from build123d import *

# Parameters (mm, degrees)
SKETCH3_R             = 2.5
SKETCH3_R_2           = 1.5
BOSS_EXTRUDE2_DEPTH   = 14
BOSS_EXTRUDE2_2_DEPTH = 14
BOSS_EXTRUDE2_3_DEPTH = 14
BOSS_EXTRUDE2_4_DEPTH = 14
BOSS_EXTRUDE3_DEPTH   = 1.5
SKETCH5_R             = 1.5
CUT_EXTRUDE1_DEPTH    = 1.5
CUT_EXTRUDE2_DEPTH    = 1.5


with BuildPart() as part:
    # Sketch3 → Boss-Extrude2 (new body)
    with BuildSketch(Plane(origin=(0, 0, 0), x_dir=(1, 0, 0), z_dir=(0, 1, 0))):
        with Locations((-31, 18)):
            Circle(SKETCH3_R)
        with Locations((-31, 18)):
            Circle(SKETCH3_R_2, mode=Mode.SUBTRACT)
    extrude(amount=BOSS_EXTRUDE2_DEPTH)



with BuildPart() as body_2:
    # Sketch3 → Boss-Extrude2 2 (new body)
    with BuildSketch(Plane(origin=(0, 0, 0), x_dir=(1, 0, 0), z_dir=(0, 1, 0))):
        with Locations((31, 18)):
            Circle(SKETCH3_R)
        with Locations((31, 18)):
            Circle(SKETCH3_R_2, mode=Mode.SUBTRACT)
    extrude(amount=BOSS_EXTRUDE2_2_DEPTH)


with BuildPart() as body_3:
    # Sketch3 → Boss-Extrude2 3 (new body)
    with BuildSketch(Plane(origin=(0, 0, 0), x_dir=(1, 0, 0), z_dir=(0, 1, 0))):
        with Locations((31, -18)):
            Circle(SKETCH3_R)
        with Locations((31, -18)):
            Circle(SKETCH3_R_2, mode=Mode.SUBTRACT)
    extrude(amount=BOSS_EXTRUDE2_3_DEPTH)


with BuildPart() as body_4:
    # Sketch3 → Boss-Extrude2 4 (new body)
    with BuildSketch(Plane(origin=(0, 0, 0), x_dir=(1, 0, 0), z_dir=(0, 1, 0))):
        with Locations((-31, -18)):
            Circle(SKETCH3_R)
        with Locations((-31, -18)):
            Circle(SKETCH3_R_2, mode=Mode.SUBTRACT)
    extrude(amount=BOSS_EXTRUDE2_4_DEPTH)


with BuildPart() as part_1:
    add(part.part)

    add(body_2.part)  # Boss-Extrude3 merges body 2

    add(body_3.part)  # Boss-Extrude3 merges body 3

    add(body_4.part)  # Boss-Extrude3 merges body 4
    # Sketch4 → Boss-Extrude3 (add)
    with BuildSketch(Plane.XZ):
        with BuildLine():
            Line((-31, 20.5), (31, 20.5))
            ThreePointArc((31, 20.5), (32.767766953, 19.767766953), (33.5, 18))
            Line((33.5, 18), (33.5, -18))
            ThreePointArc((33.5, -18), (32.767766953, -19.767766953), (31, -20.5))
            Line((31, -20.5), (-31, -20.5))
            ThreePointArc((-31, -20.5), (-32.767766953, -19.767766953), (-33.5, -18))
            Line((-33.5, -18), (-33.5, 18))
            ThreePointArc((-33.5, 18), (-32.767766953, 19.767766953), (-31, 20.5))
        make_face()
    extrude(amount=BOSS_EXTRUDE3_DEPTH)

    # Sketch5 → Cut-Extrude1 (cut)
    with BuildSketch(Plane(origin=(0, 0, 0), x_dir=(1, 0, 0), z_dir=(0, 1, 0))):
        with Locations((31, 18)):
            Circle(SKETCH5_R)
        with Locations((-31, 18)):
            Circle(SKETCH5_R)
        with Locations((-31, -18)):
            Circle(SKETCH5_R)
        with Locations((31, -18)):
            Circle(SKETCH5_R)
    extrude(amount=-CUT_EXTRUDE1_DEPTH, mode=Mode.SUBTRACT)

    # Sketch6 → Cut-Extrude2 (cut)
    with BuildSketch(Plane(origin=(0, 0, 0), x_dir=(1, 0, 0), z_dir=(0, 1, 0))):
        with BuildLine():
            Line((-23.5, 10), (-23.5, -10))
            ThreePointArc((-23.5, -10), (-25, -11.5), (-26.5, -10))
            Line((-26.5, -10), (-26.5, 10))
            ThreePointArc((-26.5, 10), (-25, 11.5), (-23.5, 10))
        make_face()
        with BuildLine():
            Line((-13.5, 10), (-13.5, -10))
            ThreePointArc((-13.5, -10), (-15, -11.5), (-16.5, -10))
            Line((-16.5, -10), (-16.5, 10))
            ThreePointArc((-16.5, 10), (-15, 11.5), (-13.5, 10))
        make_face()
        with BuildLine():
            Line((-3.5, 10), (-3.5, -10))
            ThreePointArc((-3.5, -10), (-5, -11.5), (-6.5, -10))
            Line((-6.5, -10), (-6.5, 10))
            ThreePointArc((-6.5, 10), (-5, 11.5), (-3.5, 10))
        make_face()
        with BuildLine():
            Line((6.5, 10), (6.5, -10))
            ThreePointArc((6.5, -10), (5, -11.5), (3.5, -10))
            Line((3.5, -10), (3.5, 10))
            ThreePointArc((3.5, 10), (5, 11.5), (6.5, 10))
        make_face()
        with BuildLine():
            Line((16.5, 10), (16.5, -10))
            ThreePointArc((16.5, -10), (15, -11.5), (13.5, -10))
            Line((13.5, -10), (13.5, 10))
            ThreePointArc((13.5, 10), (15, 11.5), (16.5, 10))
        make_face()
        with BuildLine():
            Line((26.5, 10), (26.5, -10))
            ThreePointArc((26.5, -10), (25, -11.5), (23.5, -10))
            Line((23.5, -10), (23.5, 10))
            ThreePointArc((23.5, 10), (25, 11.5), (26.5, 10))
        make_face()
    extrude(amount=-CUT_EXTRUDE2_DEPTH, mode=Mode.SUBTRACT)


solid = part_1.part
Here's how the part is built. I have some questions about the finished solid (model axes, mm). A direction names the side the tool comes from. Round coordinates to 2 decimals unless told otherwise and drop trailing zeros. Order: outer loops, then holes, each group sorted by start corner. A loop starts at its lowest first (then second) coordinate and runs counter-clockwise, first axis right, second up. Notation, with made-up numbers: (24.5, 5.5) -> (50.5, 5.5) arc R13 ccw to (50.5, 26.5) -> close; hole circle Ø1 at (-9, 58.5). An arc over 180 degrees is marked (long way). Return JSON: item names as keys, results as strings.
Q1. If we section it at B-B on y = 3.25: List the corners of the cut face in (x, z) for me.
Filled sheet:
{"outline": "circle Ø5 at (-31, -18); circle Ø5 at (-31, 18); circle Ø5 at (31, -18); circle Ø5 at (31, 18); hole circle Ø3 at (-31, -18); hole circle Ø3 at (-31, 18); hole circle Ø3 at (31, -18); hole circle Ø3 at (31, 18)"}
Q2. If we mould it in two halves opening along X, with no side actions, what happens to faces 4 (the flat face through (-6.5, -1, 0)), 5 (the flat face through (0, -1, -20.5))? For each: released by +X, released by -X, zero draft, split by the parting line, or undercut.
Filled sheet:
{"face 4": "undercut", "face 5": "zero draft"}
Q3. If we section it at D-D on z = -14.5: List the corners of the cut face in (x, y) for me, plus the area to 4 significant figures.
Filled sheet:
{"outline": "(-33.5, -1.5) -> (33.5, -1.5) -> (33.5, 0) -> (-33.5, 0) -> close", "area": "100.5 mm^2"}
Q4. If we section it at C-C on x = 15: List the corners of the cut face in (y, z) for me, plus the area to 3 significant figures.
Filled sheet:
{"outline": "(-1.5, -20.5) -> (0, -20.5) -> (0, -11.5) -> (-1.5, -11.5) -> close; (-1.5, 11.5) -> (0, 11.5) -> (0, 20.5) -> (-1.5, 20.5) -> close", "area": "27.0 mm^2"}
Q5. If we section it at A-A on z = -4.5: List the corners of the cut face in (x, y) for me.
Filled sheet:
{"outline": "(-33.5, -1.5) -> (-26.5, -1.5) -> (-26.5, 0) -> (-33.5, 0) -> close; (-23.5, -1.5) -> (-16.5, -1.5) -> (-16.5, 0) -> (-23.5, 0) -> close; (-13.5, -1.5) -> (-6.5, -1.5) -> (-6.5, 0) -> (-13.5, 0) -> close; (-3.5, -1.5) -> (3.5, -1.5) -> (3.5, 0) -> (-3.5, 0) -> close; (6.5, -1.5) -> (13.5, -1.5) -> (13.5, 0) -> (6.5, 0) -> close; (16.5, -1.5) -> (23.5, -1.5) -> (23.5, 0) -> (16.5, 0) -> close; (26.5, -1.5) -> (33.5, -1.5) -> (33.5, 0) -> (26.5, 0) -> close"}
Q6. For pin 1 Ø1.8 at (x, z) = (-31, -18) entering from +Y; pin 2 Ø4 at (x, z) = (14.5, 11.5) entering from +Y; pin 3 Ø3 at (y, z) = (6.5, -16) entering from -X, each with a flat end and sliding along its axis, tell me the tip position at first contact or that it passes through.
Filled sheet:
{"pin 1": "passes through", "pin 2": "stops at y = 0", "pin 3": "stops at x = -33.45"}
Q7. Which directions (+Z, -Z, +X, -X, +Y, -Y) give clear straight access to the entire face, cutting with the end or side of a thin tool? Please do faces 1 (the flat face through (0, 0, 0)), 2 (the flat face through (33, 14, -18)), 3 (the cylindrical face through (-25, -0.7, -11.5)).
Filled sheet:
{"face 1": "+Y", "face 2": "+Z, -Z, +X, -X, +Y", "face 3": "+Y, -Y"}
Q8. I need wall thicknesses on line 1 along Z through (x, y) = (31, -0.9); line 2 along X through (y, z) = (7.25, 18); line 3 along X through (y, z) = (-1.1, -18). Which ranges of each line are inside material? Lowest first, please. Write a range as from..to.
Filled sheet:
{"line 1": "z = -20.5..-19.5, -16.5..16.5, 19.5..20.5", "line 2": "x = -33.5..-32.5, -29.5..-28.5, 28.5..29.5, 32.5..33.5", "line 3": "x = -33.5..-32.5, -29.5..29.5, 32.5..33.5"}
